Work out the finished part from the listing and answer in its coordinate system (mm). Face numbers are marked on the shaded views. A direction names the side the tool comes from. Give positions to 0.01 mm unless a question says otherwise; leave off trailing zeros. Loops run counter-clockwise (first coordinate to the right, second up) from the corner with the lowest first, then second, coordinate; pieces in that order, holes last. Notation, with made-up numbers: (49, 33) - (71, 33) arc R26 ccw to (71, 65) - close; hole circle Ø2 at (-3.75, 36.25). An arc over 180 degrees is marked (long way). Use CSV: the item, a comma, the result in double quotes.
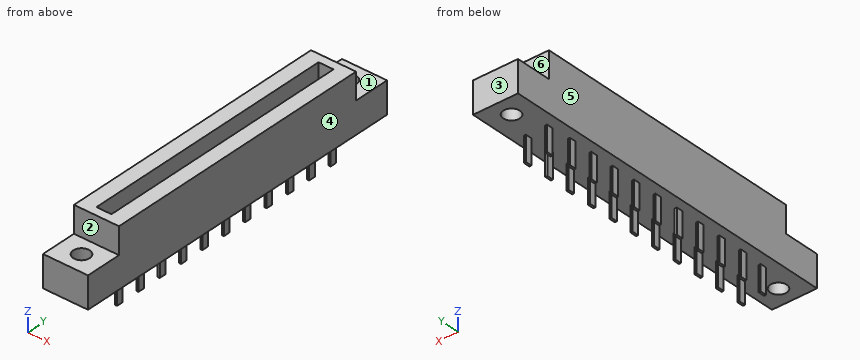
from build123d import *

# Parameters (mm, degrees)
SKETCH_1_W          = 9
SKETCH_1_H          = 70
EXTRUDE_1_DEPTH     = 6.3
SKETCH_2_W          = 9
SKETCH_2_H          = 55.5
EXTRUDE_2_DEPTH     = 5.3
SKETCH_3_R          = 1.65
CUT_EXTRUDE_1_DEPTH = 15.3
SKETCH_4_W          = 0.410265385
SKETCH_4_H          = 1.299173718
EXTRUDE_3_DEPTH     = 5
SKETCH_5_W          = 3
SKETCH_5_H          = 52
CUT_EXTRUDE_2_DEPTH = 8


with BuildPart() as part:
    # 草图1 → 拉伸1 (new body)
    with BuildSketch(Plane.XY):
        Rectangle(SKETCH_1_W, SKETCH_1_H)
    extrude(amount=EXTRUDE_1_DEPTH)

    # 草图2 → 拉伸2 (add)
    with BuildSketch(Plane.XY.offset(6.3)):
        Rectangle(SKETCH_2_W, SKETCH_2_H)
    extrude(amount=EXTRUDE_2_DEPTH)

    # 草图3 → 切除-拉伸1 (cut)
    with BuildSketch(Plane.XY.offset(6.3)):
        with Locations((0, 31.25)):
            Circle(SKETCH_3_R)
        with Locations((0, -31.25)):
            Circle(SKETCH_3_R)
    extrude(amount=-CUT_EXTRUDE_1_DEPTH, mode=Mode.SUBTRACT)

    # 草图4 → 拉伸3 (add)
    with BuildSketch(Plane(origin=(0, 0, 0), x_dir=(-1, 0, 0), z_dir=(0, 0, -1))):
        with Locations((2.113574837, 25)):
            Rectangle(SKETCH_4_W, SKETCH_4_H)
        with Locations((-2.113574837, 25)):
            Rectangle(SKETCH_4_W, SKETCH_4_H)
        with Locations((2.428938656, 20)):
            Rectangle(SKETCH_4_W, SKETCH_4_H)
        with Locations((-2.113574837, 20)):
            Rectangle(SKETCH_4_W, SKETCH_4_H)
        with Locations((2.428938656, 15)):
            Rectangle(SKETCH_4_W, SKETCH_4_H)
        with Locations((-2.113574837, 15)):
            Rectangle(SKETCH_4_W, SKETCH_4_H)
        with Locations((2.428938656, 10)):
            Rectangle(SKETCH_4_W, SKETCH_4_H)
        with Locations((-2.113574837, 10)):
            Rectangle(SKETCH_4_W, SKETCH_4_H)
        with Locations((2.428938656, 5)):
            Rectangle(SKETCH_4_W, SKETCH_4_H)
        with Locations((-2.113574837, 5)):
            Rectangle(SKETCH_4_W, SKETCH_4_H)
        with Locations((2.428938656, 0)):
            Rectangle(SKETCH_4_W, SKETCH_4_H)
        with Locations((-2.113574837, 0)):
            Rectangle(SKETCH_4_W, SKETCH_4_H)
        with Locations((-2.113574837, -5)):
            Rectangle(SKETCH_4_W, SKETCH_4_H)
        with Locations((2.428938656, -5)):
            Rectangle(SKETCH_4_W, SKETCH_4_H)
        with Locations((-2.113574837, -10)):
            Rectangle(SKETCH_4_W, SKETCH_4_H)
        with Locations((2.428938656, -10)):
            Rectangle(SKETCH_4_W, SKETCH_4_H)
        with Locations((-2.113574837, -15)):
            Rectangle(SKETCH_4_W, SKETCH_4_H)
        with Locations((2.428938656, -15)):
            Rectangle(SKETCH_4_W, SKETCH_4_H)
        with Locations((-2.113574837, -20)):
            Rectangle(SKETCH_4_W, SKETCH_4_H)
        with Locations((2.428938656, -20)):
            Rectangle(SKETCH_4_W, SKETCH_4_H)
        with Locations((2.113574837, -25)):
            Rectangle(SKETCH_4_W, SKETCH_4_H)
        with Locations((-2.113574837, -25)):
            Rectangle(SKETCH_4_W, SKETCH_4_H)
    extrude(amount=EXTRUDE_3_DEPTH)

    # 草图5 → 切除-拉伸2 (cut)
    with BuildSketch(Plane.XY.offset(11.6)):
        Rectangle(SKETCH_5_W, SKETCH_5_H)
    extrude(amount=-CUT_EXTRUDE_2_DEPTH, mode=Mode.SUBTRACT)


solid = part.part
Item 1: For the marked faces 1, 2 and 3, determine the directions among +Z, -Z, +X, -X, +Y, -Y from which every point of the face is accessible in a straight line to the end or side of a thin tool.
Determined:
face 1,"+Z, +X, -X, +Y"
face 2,"+Z, +X, -X, -Y"
face 3,"+Z, -Z, +X, -X, +Y"
Item 2: A cutting plane is placed at C-C on z = 9.5. Determine the outline of the cut face in (x, y).
Determined:
outline,"(-4.5, -27.75) - (4.5, -27.75) - (4.5, 27.75) - (-4.5, 27.75) - close; hole (-1.5, -26) - (1.5, -26) - (1.5, 26) - (-1.5, 26) - close"
Item 3: Find the intervals of material crossed by line 1 (Y direction, x = 0, z = 4.25); line 2 (Y direction, x = 0, z = 7.5); line 3 (X direction, y = 20.5, z = 11), in increasing order.
Determined:
line 1,"y = -35 to -32.9, -29.6 to -26, 26 to 29.6, 32.9 to 35"
line 2,"y = -27.75 to -26, 26 to 27.75"
line 3,"x = -4.5 to -1.5, 1.5 to 4.5"
Item 4: Given P1, Ø1.4, axis at y = 25, z = -1.5, coming from the +X side; P2, Ø4.5, axis at x = 0, y = 31.25, coming from the +Z side; P3, Ø1.4, axis at y = -5, z = -3.5, coming from the -X side, each flat-ended and moving along its own axis, determine where each tip first touches the part or whether it passes through.
Determined:
P1,"stops at x = 2.32"
P2,"stops at z = 6.3"
P3,"stops at x = -2.63"
Item 5: The mould has two halves that part along X. Classify the marked faces 4, 5 and 6: pulls with the +X half, pulls with the -X half, needs draft (parallel to the pull), parting line crosses it, or undercut.
Determined:
face 4,"pulls with the +X half"
face 5,"pulls with the -X half"
face 6,"needs draft"
Item 6: A cutting plane is placed at A-A on y = -31.25. Determine the outline of the cut face in (x, z), and give its area (3 significant figures).
Determined:
outline,"(-4.5, 0) - (-1.65, 0) - (-1.65, 6.3) - (-4.5, 6.3) - close; (1.65, 0) - (4.5, 0) - (4.5, 6.3) - (1.65, 6.3) - close"
area,"35.9 mm²"
Item 7: A cutting plane is placed at D-D on y = 17. Determine the outline of the cut face in (x, z), and give its area (3 significant figures).
Determined:
outline,"(-4.5, 0) - (4.5, 0) - (4.5, 11.6) - (1.5, 11.6) - (1.5, 3.6) - (-1.5, 3.6) - (-1.5, 11.6) - (-4.5, 11.6) - close"
area,"80.4 mm²"
Item 8: A cutting plane is placed at B-B on x = 0. Determine the outline of the cut face in (y, z).
Determined:
outline,"(-35, 0) - (-32.9, 0) - (-32.9, 6.3) - (-35, 6.3) - close; (-29.6, 0) - (29.6, 0) - (29.6, 6.3) - (27.75, 6.3) - (27.75, 11.6) - (26, 11.6) - (26, 3.6) - (-26, 3.6) - (-26, 11.6) - (-27.75, 11.6) - (-27.75, 6.3) - (-29.6, 6.3) - close; (32.9, 0) - (35, 0) - (35, 6.3) - (32.9, 6.3) - close"
